Could you check a few things on this model? Use its own coordinates, in mm. A direction names the side the tool comes from. Coordinates: 2 decimals unless noted, no trailing zeros. Loops run counter-clockwise (first coordinate to the right, second up) from the corner with the lowest first, then second, coordinate; pieces in that order, holes last. Notation, with made-up numbers: (73, -8.5) -> (126, -8.5) arc R16 ccw to (126, 9.5) -> close; hole circle Ø11 at (42, -8). An arc over 180 degrees is marked (long way). One line per question, with ' | ' between items. Start each with the question number.
(1) If we mould it in two halves opening along Z, with no side actions, what happens to faces 1 (the face through (0.07, 7.15, 31.99)), 2 (the face through (-11.923, 3.755, -73.95)), 3 (the face through (-0.07, 1.08, 20.12))? For each: pulls with the +Z half, pulls with the -Z half, needs draft (parallel to the pull), parting line crosses it, or undercut.
(2) Suppose I cut it at B-B (z = -63). Please give me the cut outline in (x, y).
(3) Suppose I cut it at C-C (x = 20). Please give me the cut outline in (y, z), plus the area to 3 significant figures.
(4) Suppose I cut it at D-D (y = 18.5). Please give me the cut outline in (x, z).
(5) If I drill on line 1 along Z through (x, y) = (1, 0); line 2 along Z through (x, y) = (19, 5.5); line 3 along Y through (x, z) = (0.5, -31.5), over which ranges is the centre line in solid material (lowest first)?
(6) Which directions (+Z, -Z, +X, -X, +Y, -Y) give clear straight access to the entire face, cutting with the end or side of a thin tool? Please do faces 4 (the face through (-11.5, 5.9, 0)), 5 (the face through (-5, -0.1, 19.5)), 6 (the face through (0, -10, 17)), 7 (the face through (5, -0.1, 19.5)), 8 (the face through (0, 10, 17)).
(7) I'm going to push flat-ended pins straight in: pin 1 Ø4 at (x, z) = (-3.5, -26) entering from +Y; pin 2 Ø22 at (y, z) = (3.5, 27) entering from -X; pin 3 Ø3 at (x, z) = (0, 19) entering from -Y. Where does each tip first touch, or does it pass through?
```python
from build123d import *

# Parameters (mm, degrees)
SKETCH2_R           = 25
BOSS_EXTRUDE2_DEPTH = 10
SKETCH3_W           = 10
SKETCH3_H           = 20
BOSS_EXTRUDE3_DEPTH = 25
SKETCH4_R           = 5
CUT_EXTRUDE1_DEPTH  = 20
FILLET1_R           = 10
SKETCH5_R           = 12.5
BOSS_EXTRUDE4_DEPTH = 150


with BuildPart() as part:
    # Sketch2 → Boss-Extrude2 (new body)
    with BuildSketch(Plane.XY):
        Circle(SKETCH2_R)
    extrude(amount=BOSS_EXTRUDE2_DEPTH)

    # Sketch3 → Boss-Extrude3 (add)
    with BuildSketch(Plane.XY.offset(10)):
        Rectangle(SKETCH3_W, SKETCH3_H)
    extrude(amount=BOSS_EXTRUDE3_DEPTH)

    # Sketch4 → Cut-Extrude1 (cut)
    with BuildSketch(Plane.ZY.offset(5)):
        with Locations(Location((25, 0, 0), (0, 0, 270))):
            Circle(SKETCH4_R)
    extrude(amount=-CUT_EXTRUDE1_DEPTH, mode=Mode.SUBTRACT)

    # Fillet1
    fillet1_edges = [part.edges().sort_by_distance(p)[0] for p in [
        (0, -10, 35),
        (0, 10, 35),
    ]]
    fillet(fillet1_edges, radius=FILLET1_R - 0.0001)  # a hair under: the kernel refuses the full size

    # Sketch5 → Boss-Extrude4 (add)
    with BuildSketch(Plane(origin=(0, 0, 0), x_dir=(-1, 0, 0), z_dir=(0, 0, -1))):
        Circle(SKETCH5_R)
    extrude(amount=BOSS_EXTRUDE4_DEPTH)


solid = part.part
```
Checks:
1) face 1: pulls with the +Z half | face 2: needs draft | face 3: undercut
2) outline: circle Ø25 at (0, 0)
3) outline: (-15, 0) -> (15, 0) -> (15, 10) -> (-15, 10) -> close | area: 300 mm^2
4) outline: (-16.82, 0) -> (16.82, 0) -> (16.82, 10) -> (-16.82, 10) -> close
5) line 1: z = -150 to 20, 30 to 35 | line 2: z = 0 to 10 | line 3: y = -12.49 to 12.49
6) face 4: -Z | face 5: +Z, -X, +Y, -Y | face 6: +Z, +X, -X, -Y | face 7: +Z, +X, +Y, -Y | face 8: +Z, +X, -X, +Y
7) pin 1: stops at y = 12.41 | pin 2: stops at x = -5 | pin 3: stops at y = -10
